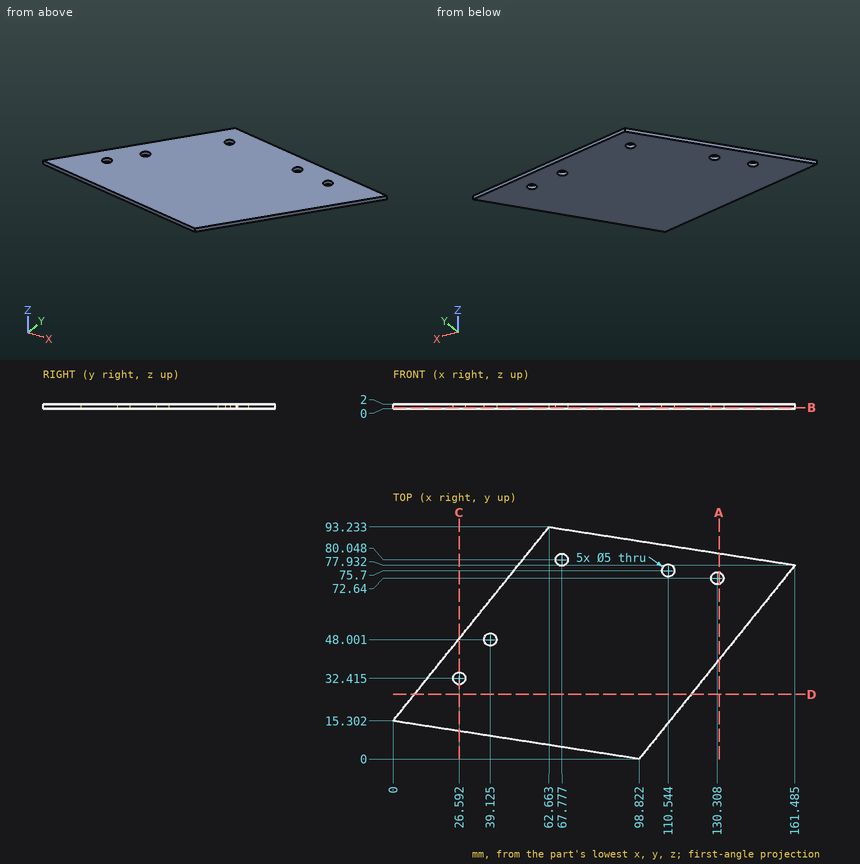
The drawing under review shows one solid part. Ordinate dimensions are in mm from its lowest x, y, z. Give positions to 0.01 mm unless a question says otherwise; leave off trailing zeros. Write each loop counter-clockwise with the first axis right and the second up, starting at its lowest first coordinate (ties: lowest second). Pieces come first, ordered by that corner, then holes. Notation, with made-up numbers: (7, 84.5) - (22, 84.5) arc R13 ccw to (22, 94.5) - close; hole circle Ø6 at (33, 36). An arc over 180 degrees is marked (long way). Answer in a Markdown table with one row per item. Add a question column.
1. Wall thickness on line 1 along X through (y, z) = (32.5, 1) (1 decimal); line 2 along Y through (x, z) = (109.5, 1.5) (1 decimal); line 3 along X through (y, z) = (72, 0.4) (1 decimal): over which ranges is each line inside the solid? List them lowest first. Write a range as [from, to].
2. We need section B-B on z = 0.55. Write out the cut boundary in (x, y) (1 decimal).
3. We need section A-A on x = 131. Write out the cut boundary in (y, z).
4. Insertion check: P1, Ø3, axis at x = 110.54, y = 75.7, coming from the -Z side. The pin has a flat end and moves straight along its axis. Give the tip position at first contact, or say it passes through.
5. We need section D-D on y = 26. Write out the cut boundary in (x, z), then the cut area to 3 significant figures.
6. We need section C-C on x = 26.5. Write out the cut boundary in (y, z).
Ans:
| question | item | result |
|---|---|---|
| 1 | line 1 | x = [13.8, 24.1], [29.1, 125] |
| 1 | line 2 | y = [13.3, 73.4], [78, 86] |
| 1 | line 3 | x = [45.6, 127.9], [132.7, 156.7] |
| 2 | outline | (0, 15.3) - (98.8, 0) - (161.5, 77.9) - (62.7, 93.2) - close; hole circle Ø5 at (26.6, 32.4); hole circle Ø5 at (39.1, 48); hole circle Ø5 at (67.8, 80); hole circle Ø5 at (110.5, 75.7); hole circle Ø5 at (130.3, 72.6) |
| 3 | outline | (40.02, 0) - (70.24, 0) - (70.24, 2) - (40.02, 2) - close; (75.04, 0) - (82.65, 0) - (82.65, 2) - (75.04, 2) - close |
| 4 | P1 | passes through |
| 5 | outline | (8.6, 0) - (119.73, 0) - (119.73, 2) - (8.6, 2) - close |
| 5 | area | 222 mm^2 |
| 6 | outline | (11.2, 0) - (29.92, 0) - (29.92, 2) - (11.2, 2) - close; (34.91, 0) - (48.26, 0) - (48.26, 2) - (34.91, 2) - close |
